The model under review builds one solid part; all positions refer to its coordinate system, in mm. Give positions to 0.01 mm unless a question says otherwise; leave off trailing zeros. Order: outer loops, then holes, each group sorted by start corner. A loop starts at its lowest first (then second) coordinate and runs counter-clockwise, first axis right, second up.
Autodesk Inventor part; units mm, degrees
ref_plane "Work Plane2" through (0, 1.4, 0) normal (0, 1, 0) x (1, 0, 0)
ref_plane "YZ Plane" through (0, 0, 0) normal (1, 0, 0) x (0, 1, 0)
ref_plane "XZ Plane" through (0, 0, 0) normal (0, 1, 0) x (-1, 0, 0)
sketch "Sketch1" plane through (0, 0, 0) normal (0, 1, 0) x (-1, 0, 0)
  line L0 (-6, 19) -> (6, 19)
  line L1 (6, 19) -> (6, -19)
  line L2 (6, -19) -> (-6, -19)
  line L3 (-6, -19) -> (-6, 19)
  line L4 (-6, 19) -> (6, -19) construction
  line L5 (6, 19) -> (-6, -19) construction
  line L6 (5.502, -16) -> (-5.998, -16)
  line L7 (5.502, 14) -> (5.502, -16)
  line L8 (0, 19) -> (0, -19) construction
  line L9 (5.503, 14.001) -> (-5.999, 14.001)
  line L10 (-5.999, 14.001) -> (-5.999, -12.599)
  line L11 (-5.999, -12.599) -> (5.503, -12.599)
  line L12 (3.541, 12.89) -> (-4.039, 12.89)
  line L13 (-4.039, 12.89) -> (-4.039, -11.49)
  line L14 (-4.039, -11.49) -> (3.541, -11.49)
  line L15 (3.541, -11.49) -> (3.541, 12.89)
  line L16 (2.541, 11.89) -> (-3.039, 11.89)
  line L17 (-3.039, 11.89) -> (-3.039, -10.49)
  line L18 (-3.039, -10.49) -> (2.541, -10.49)
  line L19 (2.541, -10.49) -> (2.541, 11.89)
  line L20 (-0.249, 12.89) -> (-0.249, -11.49) construction
  line L21 (3.541, 0.7) -> (-4.039, 0.7) construction
  circle A0 centre (-3.81, 17.04) radius 0.5
  circle A1 centre (-1.27, 17.04) radius 0.5
  circle A2 centre (1.27, 17.04) radius 0.5
  circle A3 centre (3.81, 17.04) radius 0.5
  line L22 (3.041, -13.8) -> (-3.539, -13.8)
  line L23 (-3.539, -13.8) -> (-3.539, -14.8)
  line L24 (-3.539, -14.8) -> (3.041, -14.8)
  line L25 (3.041, -14.8) -> (3.041, -13.8)
  line L26 (5.502, 14) -> (-5.998, 14)
  line L27 (5.503, -12.599) -> (5.503, 14.001)
  line L28 (-5.998, 14) -> (-5.998, -16)
  point P0 (0, 0)
  dimension "d0" = 12
  dimension "d1" = 38
  dimension "d2" = 3
  dimension "d3" = 30
  dimension "d5" = 26.6
  dimension "d6" = 7.58
  dimension "d7" = 24.38
  dimension "d8" = 5.58
  dimension "d9" = 22.38
  dimension "d10" = 1.96
  dimension "d11" = 7.51
  dimension "d13" = 2.19
  dimension "d14" = 1.96
  dimension "d15" = 1
  dimension "d18" = 2.54
  dimension "d27" = 1
  dimension "d28" = 1.2
  dimension "d32" = 0.001
  dimension "d33" = 0.001
  dimension "d34" = 0.001
  dimension "d35" = 11.5
  dimension "d36" = 0.001
extrude "Extrusion1" add sketch "Sketch1" against normal blind 1.2 contours L0 L1 L2 L3 L6 L7 L9 | L9 L7 L11 L3 | L11 L7 L6 L3 | L15 L14 L13 L12 | L19 L18 L17 L16 | L25 L24 L23 L22
extrude "Extrusion2" add sketch "Sketch1" along normal blind 0.5 contours L9 L7 L11 L3 | L15 L14 L13 L12 | L19 L18 L17 L16 | L25 L24 L23 L22
sketch "Sketch2" plane through (0, 0.5, 0) normal (0, 1, 0) x (1, 0, 0)
  line L0 (-5.502, -14) -> (-5.502, 16)
  line L1 (-5.502, 16) -> (5.998, 16)
  line L2 (-5.502, -14) -> (5.998, -14)
  line L3 (5.998, -14) -> (5.998, 16)
  line L4 (-3.541, -12.89) -> (4.039, -12.89)
  line L5 (-3.541, 11.49) -> (-3.541, -12.89)
  line L6 (4.039, -12.89) -> (4.039, 11.49)
  line L7 (4.039, 11.49) -> (-3.541, 11.49)
  point P0 (0, 0)
extrude "Extrusion3" add sketch "Sketch2" along normal blind 0.5 contours L0 L1 L3 L2 | L5 L7 L6 L4
sketch "Sketch3" plane through (0, 1, 0) normal (0, 1, 0) x (1, 0, 0)
  line L0 (-2.541, -11.89) -> (3.039, -11.89)
  line L1 (-2.541, 10.49) -> (-2.541, -11.89)
  line L2 (3.039, -11.89) -> (3.039, 10.49)
  line L3 (3.039, 10.49) -> (-2.541, 10.49)
  point P0 (0, 0)
extrude "Extrusion4" add sketch "Sketch3" along normal blind 0.2
extrude "Extrusion5" cut sketch "Sketch2" against normal blind 0.5 contours L5 L7 L6 L4
fillet "Fillet1" radius 1 4 edges at (-3.541, 0.25, 12.89) (4.039, 0.25, -11.49) (-3.541, 0.25, -11.49) (4.039, 0.25, 12.89)
sketch "Sketch4" plane through (0, -1.2, 0) normal (0, 1, 0) x (1, 0, 0)
  line L0 (2.785, -15.895) -> (2.585, -16.095)
  line L1 (2.585, -16.095) -> (2.585, -17.985)
  line L2 (2.585, -17.985) -> (2.785, -18.185)
  line L3 (2.785, -18.185) -> (4.835, -18.185)
  line L4 (4.835, -18.185) -> (5.035, -17.985)
  line L5 (5.035, -17.985) -> (5.035, -16.095)
  line L6 (5.035, -16.095) -> (4.835, -15.895)
  line L7 (4.835, -15.895) -> (2.785, -15.895)
  line L8 (3.81, -18.185) -> (3.81, -15.895) construction
  line L9 (2.585, -17.04) -> (5.035, -17.04) construction
  circle A0 centre (3.81, -17.04) radius 0.5 construction
  line L10 (3.51, -17.34) -> (4.11, -17.34)
  line L11 (4.11, -17.34) -> (4.11, -16.74)
  line L12 (4.11, -16.74) -> (3.51, -16.74)
  line L13 (3.51, -16.74) -> (3.51, -17.34)
  line L14 (3.51, -17.34) -> (4.11, -16.74) construction
  line L15 (4.11, -17.34) -> (3.51, -16.74) construction
  line L16 (6, -19) -> (-6, -19) construction
  line L17 (0.245, -15.895) -> (0.045, -16.095)
  line L18 (0.045, -16.095) -> (0.045, -17.985)
  line L19 (0.045, -17.985) -> (0.245, -18.185)
  line L20 (0.245, -18.185) -> (2.295, -18.185)
  line L21 (2.295, -18.185) -> (2.495, -17.985)
  line L22 (2.495, -17.985) -> (2.495, -16.095)
  line L23 (2.495, -16.095) -> (2.295, -15.895)
  line L24 (2.295, -15.895) -> (0.245, -15.895)
  line L25 (1.27, -18.185) -> (1.27, -15.895) construction
  line L26 (0.045, -17.04) -> (2.495, -17.04) construction
  circle A1 centre (1.27, -17.04) radius 0.5 construction
  line L27 (0.97, -17.34) -> (1.57, -17.34)
  line L28 (1.57, -17.34) -> (1.57, -16.74)
  line L29 (1.57, -16.74) -> (0.97, -16.74)
  line L30 (0.97, -16.74) -> (0.97, -17.34)
  line L31 (0.97, -17.34) -> (1.57, -16.74) construction
  line L32 (1.57, -17.34) -> (0.97, -16.74) construction
  line L33 (-2.295, -15.895) -> (-2.495, -16.095)
  line L34 (-2.495, -16.095) -> (-2.495, -17.985)
  line L35 (-2.495, -17.985) -> (-2.295, -18.185)
  line L36 (-2.295, -18.185) -> (-0.245, -18.185)
  line L37 (-0.245, -18.185) -> (-0.045, -17.985)
  line L38 (-0.045, -17.985) -> (-0.045, -16.095)
  line L39 (-0.045, -16.095) -> (-0.245, -15.895)
  line L40 (-0.245, -15.895) -> (-2.295, -15.895)
  line L41 (-1.27, -18.185) -> (-1.27, -15.895) construction
  line L42 (-2.495, -17.04) -> (-0.045, -17.04) construction
  circle A2 centre (-1.27, -17.04) radius 0.5 construction
  line L43 (-1.57, -17.34) -> (-0.97, -17.34)
  line L44 (-0.97, -17.34) -> (-0.97, -16.74)
  line L45 (-0.97, -16.74) -> (-1.57, -16.74)
  line L46 (-1.57, -16.74) -> (-1.57, -17.34)
  line L47 (-1.57, -17.34) -> (-0.97, -16.74) construction
  line L48 (-0.97, -17.34) -> (-1.57, -16.74) construction
  line L49 (-4.835, -15.895) -> (-5.035, -16.095)
  line L50 (-5.035, -16.095) -> (-5.035, -17.985)
  line L51 (-5.035, -17.985) -> (-4.835, -18.185)
  line L52 (-4.835, -18.185) -> (-2.785, -18.185)
  line L53 (-2.785, -18.185) -> (-2.585, -17.985)
  line L54 (-2.585, -17.985) -> (-2.585, -16.095)
  line L55 (-2.585, -16.095) -> (-2.785, -15.895)
  line L56 (-2.785, -15.895) -> (-4.835, -15.895)
  line L57 (-3.81, -18.185) -> (-3.81, -15.895) construction
  line L58 (-5.035, -17.04) -> (-2.585, -17.04) construction
  circle A3 centre (-3.81, -17.04) radius 0.5 construction
  line L59 (-4.11, -17.34) -> (-3.51, -17.34)
  line L60 (-3.51, -17.34) -> (-3.51, -16.74)
  line L61 (-3.51, -16.74) -> (-4.11, -16.74)
  line L62 (-4.11, -16.74) -> (-4.11, -17.34)
  line L63 (-4.11, -17.34) -> (-3.51, -16.74) construction
  line L64 (-3.51, -17.34) -> (-4.11, -16.74) construction
  circle A4 centre (-3.81, -17.04) radius 0.5 construction
  circle A5 centre (-1.27, -17.04) radius 0.5 construction
  circle A6 centre (1.27, -17.04) radius 0.5 construction
  point P0 (0, 0)
  point P1 (-1.27, -17.04)
  dimension "d43" = 2.05
  dimension "d46" = 1.89
  dimension "d47" = 0.2828
  dimension "d48" = 45
  dimension "d49" = 0.6
  dimension "d50" = 0.6
  dimension "d53" = 135
  dimension "d54" = 135
  dimension "d55" = 135
  dimension "d56" = 2.05
  dimension "d57" = 1.89
  dimension "d58" = 0.2828
  dimension "d59" = 45
  dimension "d60" = 0.6
  dimension "d61" = 0.6
  dimension "d62" = 135
  dimension "d63" = 135
  dimension "d64" = 135
  dimension "d65" = 2.05
  dimension "d66" = 1.89
  dimension "d67" = 0.2828
  dimension "d68" = 45
  dimension "d69" = 0.6
  dimension "d70" = 0.6
  dimension "d71" = 135
  dimension "d72" = 135
  dimension "d73" = 135
  dimension "d74" = 2.05
  dimension "d75" = 1.89
  dimension "d76" = 0.2828
  dimension "d77" = 45
  dimension "d78" = 0.6
  dimension "d79" = 0.6
  dimension "d80" = 135
  dimension "d81" = 135
  dimension "d82" = 135
extrude "Extrusion6" [suppressed]
ref_plane "Work Plane2" through (0, 1.4, 0) normal (0, 1, 0) x (1, 0, 0)
sketch "Sketch5" plane through (0, 1.4, 0) normal (0, 1, 0) x (1, 0, 0)
  line L0 (4.11, -16.74) -> (4.11, -17.34)
  line L1 (4.11, -17.34) -> (3.51, -17.34)
  line L2 (3.51, -17.34) -> (3.51, -16.74)
  line L3 (3.51, -16.74) -> (4.11, -16.74)
  line L4 (1.57, -16.74) -> (1.57, -17.34)
  line L5 (0.97, -16.74) -> (1.57, -16.74)
  line L6 (1.57, -17.34) -> (0.97, -17.34)
  line L7 (0.97, -17.34) -> (0.97, -16.74)
  line L8 (-3.51, -16.74) -> (-3.51, -17.34)
  line L9 (-3.51, -17.34) -> (-4.11, -17.34)
  line L10 (-4.11, -17.34) -> (-4.11, -16.74)
  line L11 (-4.11, -16.74) -> (-3.51, -16.74)
  line L12 (-0.97, -16.74) -> (-0.97, -17.34)
  line L13 (-0.97, -17.34) -> (-1.57, -17.34)
  line L14 (-1.57, -17.34) -> (-1.57, -16.74)
  line L15 (-1.57, -16.74) -> (-0.97, -16.74)
  point P0 (0, 0)
  point P1 (4.11, 17.34)
  point P2 (4.11, 16.74)
  point P3 (3.51, 17.34)
  point P4 (3.51, 16.74)
  point P5 (1.57, 17.34)
  point P6 (1.57, 16.74)
  point P7 (0.97, 16.74)
  point P8 (0.97, 17.34)
  point P9 (-3.51, 17.34)
  point P10 (-3.51, 16.74)
  point P11 (-4.11, 17.34)
  point P12 (-4.11, 16.74)
  point P13 (-0.97, 17.34)
  point P14 (-0.97, 16.74)
  point P15 (-1.57, 17.34)
  point P16 (-1.57, 16.74)
extrude "Extrusion7" [suppressed]
properties part number "LED Screen 0.91 inch"
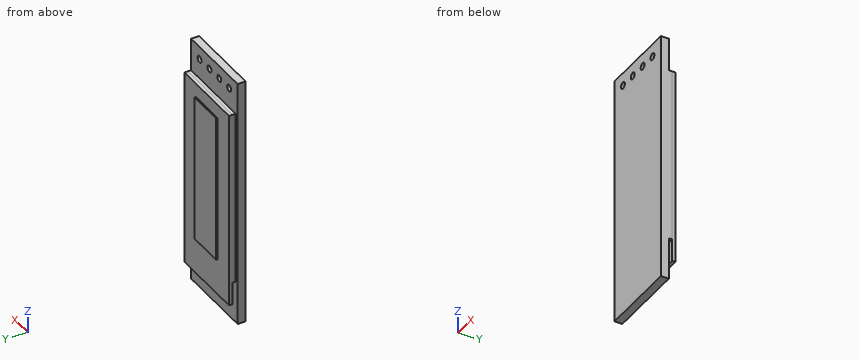
Item 1: Take a section at A-A (z = 17.04). Give the boundary of the cut face in (x, y).
Values found:
outline: (-6, -1.2) - (-4.31, -1.2) - (-4.31, 0) - (-6, 0) - close; (-3.31, -1.2) - (-1.77, -1.2) - (-1.77, 0) - (-3.31, 0) - close; (-0.77, -1.2) - (0.77, -1.2) - (0.77, 0) - (-0.77, 0) - close; (1.77, -1.2) - (3.31, -1.2) - (3.31, 0) - (1.77, 0) - close; (4.31, -1.2) - (6, -1.2) - (6, 0) - (4.31, 0) - close
Item 2: Take a section at C-C (z = -5.5). Give the boundary of the cut face in (x, y).
Values found:
outline: (-6, -1.2) - (6, -1.2) - (6, 1) - (3.04, 1) - (3.04, 1.2) - (-2.54, 1.2) - (-2.54, 1) - (-5.5, 1) - (-5.5, 0) - (-6, 0) - close; hole (-3.54, 0) - (4.04, 0) - (4.04, 0.5) - (-3.54, 0.5) - close
Item 3: Take a section at B-B (x = 1.27). Give the boundary of the cut face in (y, z), and give its area (3 significant figures).
Values found:
outline: (-1.2, -19) - (0, -19) - (0, -14.8) - (0.5, -14.8) - (0.5, -16) - (1, -16) - (1, -10.49) - (1.2, -10.49) - (1.2, 11.89) - (1, 11.89) - (1, 14) - (0, 14) - (0, 16.54) - (-1.2, 16.54) - close; (-1.2, 17.54) - (0, 17.54) - (0, 19) - (-1.2, 19) - close; hole (0, -13.8) - (0.5, -13.8) - (0.5, -12.6) - (0, -12.6) - close; hole (0, -11.49) - (0.5, -11.49) - (0.5, 12.89) - (0, 12.89) - close
area: 65.5 mm2
Item 4: For line 1 (Y direction, x = -2, z = 6); line 2 (Y direction, x = -2.25, z = 12); line 3 (Z direction, x = -1.27, y = -0.85), list the stretches that pass through material, from the lowest coordinate up.
Values found:
line 1: y = -1.2 to 0, 0.5 to 1.2
line 2: y = -1.2 to 0, 0.5 to 1
line 3: z = -19 to 16.54, 17.54 to 19
Item 5: Take a section at D-D (x = 5). Give the boundary of the cut face in (y, z), and give its area (3 significant figures).
Values found:
outline: (-1.2, -19) - (0, -19) - (0, -12.6) - (0.5, -12.6) - (0.5, -16) - (1, -16) - (1, 14) - (0, 14) - (0, 19) - (-1.2, 19) - close
area: 73.9 mm2
